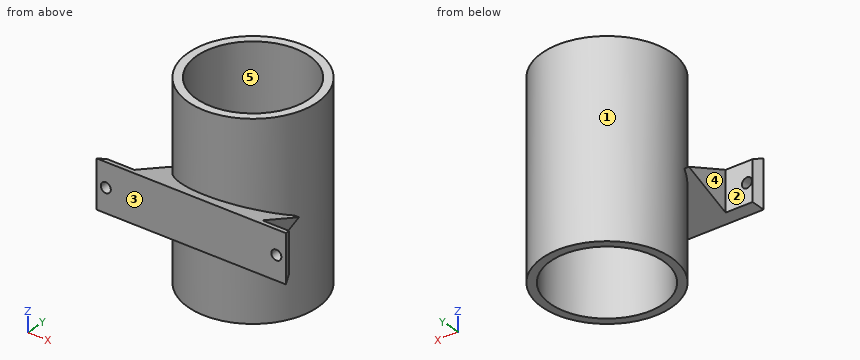
from build123d import *

# Parameters (mm, degrees)
SKETCH1_R               = 42.8625
SKETCH1_R_2             = 37.30625
BOSS_EXTRUDE1_DEPTH     = 63.5
BOSS_EXTRUDE2_START     = 34.23763648
BOSS_EXTRUDE2_DEPTH     = 13.38736352
BOSS_EXTRUDE2_START_2   = -47.625
BOSS_EXTRUDE2_2_DEPTH   = 4.7624999
BOSS_EXTRUDE2_START_3   = -63.5
BOSS_EXTRUDE2_3_DEPTH   = 127
BOSS_EXTRUDE2_START_4   = -63.5000001
BOSS_EXTRUDE2_4_DEPTH   = 127.0000002
SKETCH3_W               = 20.6375
SKETCH3_H               = 31.75
CUT_EXTRUDE1_DEPTH      = 128.485244907
F_1_4_CLEARANCE_HOLE1_D = 6.7564


with BuildPart() as part:
    # Sketch1 → Boss-Extrude1 (new, symmetric)
    with BuildSketch(Plane.XY):
        Circle(SKETCH1_R)
        Circle(SKETCH1_R_2, mode=Mode.SUBTRACT)
    extrude(amount=BOSS_EXTRUDE1_DEPTH, both=True)

    # Boss-Extrude2: read off the stored shape, not the designer's step
    # Boss-Extrude2 outline → Boss-Extrude2 (add)
    with BuildSketch(Plane.YZ.offset(BOSS_EXTRUDE2_START)):
        Polygon((-53.975, 15.875), (-53.975, -15.875), (-15.649359697, 0), align=None)
    extrude(amount=BOSS_EXTRUDE2_DEPTH)



with BuildPart() as body_2:
    # Boss-Extrude2 2 outline → Boss-Extrude2 2 (new body)
    with BuildSketch(Plane.YZ.offset(BOSS_EXTRUDE2_START_2)):
        Polygon((-53.975, 15.875), (-53.975, -15.875), (-15.649359697, 0), align=None)
    extrude(amount=BOSS_EXTRUDE2_2_DEPTH)


with BuildPart() as part_1:
    add(part.part)

    add(body_2.part)  # Boss-Extrude2 3 merges body 2
    # Boss-Extrude2 3 outline → Boss-Extrude2 3 (add)
    with BuildSketch(Plane.YZ.offset(BOSS_EXTRUDE2_START_3)):
        Polygon((-53.975, 15.875), (-53.975, -15.875), (-15.649359697, 0), align=None)
    extrude(amount=BOSS_EXTRUDE2_3_DEPTH)

    # Boss-Extrude2 4 outline → Boss-Extrude2 4 (cut)
    with BuildSketch(Plane.XY.offset(BOSS_EXTRUDE2_START_4)):
        with BuildLine():
            Line((34.57970921, -14), (-34.57970921, -14))
            ThreePointArc((-34.57970921, -14), (0, -37.30625), (34.57970921, -14))
        make_face()
        Polygon((-47.625, -15.649359697), (-46.941812844, -14), (-63.5, -14), (-63.5, -53.975), align=None)
        Polygon((63.5, -14), (46.941812844, -14), (47.625, -15.649359697), (63.5, -53.975), align=None)
    extrude(amount=BOSS_EXTRUDE2_4_DEPTH, mode=Mode.SUBTRACT)

    # Sketch3 → Cut-Extrude1 (cut, through all)
    with BuildSketch(Plane(origin=(0, -47.625, 0), x_dir=(1, 0, 0), z_dir=(0, 1, 0))):
        with Locations((-53.18125, 0)):
            Rectangle(SKETCH3_W, SKETCH3_H)
        with Locations((53.18125, 0)):
            Rectangle(SKETCH3_W, SKETCH3_H)
    extrude(amount=CUT_EXTRUDE1_DEPTH, mode=Mode.SUBTRACT)

    # 1/4 Clearance Hole1 (through all)
    with Locations(Plane(origin=(0, -47.625, 0), x_dir=(1, 0, 0), z_dir=(0, 1, 0))):
        with Locations((-57.15, 0), (57.15, 0)):
            Hole(F_1_4_CLEARANCE_HOLE1_D / 2)


solid = part_1.part
Here's how the part is built. I have some questions about the finished solid (model axes, mm). Face numbers are marked on the shaded views. A direction names the side the tool comes from. Coordinates: 2 decimals unless noted, no trailing zeros. Order: outer loops, then holes, each group sorted by start corner. A loop starts at its lowest first (then second) coordinate and runs counter-clockwise, first axis right, second up. Notation, with made-up numbers: (87.25, 58) - (137.25, 58) arc R12 cw to (137.25, 70) - close; hole circle Ø7 at (23, -4.75). An arc over 180 degrees is marked (long way). Use CSV: the item, a comma, the result in double quotes. Start each with the question number.
1. Suppose I cut it at A-A on y = 0. List the corners of the cut face in (x, z) for me, then the cut area to 3 significant figures.
2. Please list where these lines run through material, in increasing order: line 1 (X direction, y = 0, z = -11); line 2 (Y direction, x = -21.5, z = -30.5); line 3 (X direction, y = -15, z = 48). Write a range as from..to.
3. If we mould it in two halves opening along Y, with no side actions, what happens to the marked faces 3, 4 and 5? For each: +Y half, -Y half, draft (parallel to the pull), parting line (faces both ways), or undercut.
4. I'm going to push flat-ended pins straight in: pin 1 (5 mm diameter, centred on y = 8, z = 36, fed in from +X); pin 2 (13 mm diameter, centred on y = -35.5, z = 1, fed in from -X); pin 3 (3 mm diameter, centred on y = -19.5, z = 47.5, fed in from +X); pin 4 (4 mm diameter, centred on x = -57.15, z = 0, fed in from +Y). Where does each tip first touch, or does it pass through?
5. For the marked faces 1 and 2, which set-ups out of +Z, -Z, +X, -X, +Y, -Y let a thin tool reach every point of the face, with its end or its side?
6. Suppose I cut it at B-B on x = 57.15. List the corners of the cut face in (y, z) for me (3 decimals).
7. Suppose I cut it at C-C on z = 30.5. List the corners of the cut face in (x, y) for me (1 decimal), then the cut area to 3 significant figures.
8. Suppose I cut it at D-D on x = 0. List the corners of the cut face in (y, z) for me (1 decimal), then the cut area to 3 significant figures.
Output:
1,outline,"(-42.86, -63.5) - (-37.31, -63.5) - (-37.31, 63.5) - (-42.86, 63.5) - close; (37.31, -63.5) - (42.86, -63.5) - (42.86, 63.5) - (37.31, 63.5) - close"
1,area,"1,410 mm2"
2,line 1,"x = -42.86..-37.31, 37.31..42.86"
2,line 2,"y = -37.08..-30.49, 30.49..37.08"
2,line 3,"x = -40.15..-34.16, 34.16..40.15"
3,face 3,"-Y half"
3,face 4,"draft"
3,face 5,"undercut"
4,pin 1,"stops at x = 42.51"
4,pin 2,"stops at x = -42.86"
4,pin 3,"stops at x = 38.9"
4,pin 4,"passes through"
5,face 1,"none"
5,face 2,"+Z, -Z, -X, +Y"
6,outline,"(-53.975, -15.875) - (-47.625, -13.245) - (-47.625, -3.378) - (-53.975, -3.378) - close; (-53.975, 3.378) - (-47.625, 3.378) - (-47.625, 13.245) - (-53.975, 15.875) - close"
7,outline,"circle Ø85.7 at (0, 0); hole circle Ø74.6 at (0, 0)"
7,area,"1,400 mm2"
8,outline,"(-54, -15.9) - (-42.9, -11.3) - (-42.9, -63.5) - (-37.3, -63.5) - (-37.3, 63.5) - (-42.9, 63.5) - (-42.9, 11.3) - (-54, 15.9) - close; (37.3, -63.5) - (42.9, -63.5) - (42.9, 63.5) - (37.3, 63.5) - close"
8,area,"1,710 mm2"
